from build123d import *

# Parameters (mm, degrees)
SKETCH2_W           = 250
SKETCH2_H           = 30
BOSS_EXTRUDE1_DEPTH = 10
SKETCH3_W           = 5
SKETCH3_H           = 30
BOSS_EXTRUDE2_DEPTH = 10
SKETCH4_W           = 150
SKETCH4_H           = 30
BOSS_EXTRUDE3_DEPTH = 6
FILLET1_R           = 15
FILLET8_R           = 25
CHAMFER1_SIZE       = 17
FILLET3_R           = 20
FILLET5_R           = 6
FILLET6_R           = 2
FILLET7_R           = 8
SKETCH7_W           = 24
SKETCH7_H           = 24
CUT_EXTRUDE1_DEPTH  = 3


with BuildPart() as part:
    # Sketch2 → Boss-Extrude1 (new body)
    with BuildSketch(Plane(origin=(-23.43534086, 72.126562752, 0), x_dir=(0.9510565162951534, 0.3090169943749482, 0), z_dir=(-0.3090169943749481, 0.9510565162951533, 0))):
        with Locations((33.98053096, 100)):
            Rectangle(SKETCH2_W, SKETCH2_H)
    extrude(amount=-BOSS_EXTRUDE1_DEPTH)

    # Sketch3 → Boss-Extrude2 (add)
    with BuildSketch(Plane(origin=(-23.43534086, 72.126562752, 0), x_dir=(0.9510565162951534, 0.3090169943749482, 0), z_dir=(-0.3090169943749481, 0.9510565162951533, 0))):
        with Locations((-88.51946904, 100)):
            Rectangle(SKETCH3_W, SKETCH3_H)
    extrude(amount=BOSS_EXTRUDE2_DEPTH)



with BuildPart() as body_2:
    # Sketch4 → Boss-Extrude3 (new body)
    with BuildSketch(Plane(origin=(0, 0, 0), x_dir=(1, 0, 0), z_dir=(0, 1, 0))):
        with Locations((55.854299018, 100)):
            Rectangle(SKETCH4_W, SKETCH4_H)
    extrude(amount=BOSS_EXTRUDE3_DEPTH)


with BuildPart() as part_1:
    add(part.part)

    add(body_2.part)  # Loft1 merges body 2
    # Sketch6 → Loft1 section 0
    with BuildSketch(Plane(origin=(-20.345170916, 62.615997589, 0), x_dir=(0.9510565162951534, 0.3090169943749482, 0), z_dir=(0.3090169943749481, -0.9510565162951533, 0))):
        with BuildLine():
            Line((158.98053096, -85), (148.98053096, -85))
            Line((148.98053096, -85), (148.98053096, -115))
            Line((148.98053096, -115), (158.98053096, -115))
            Line((158.98053096, -115), (158.98053096, -85))
        make_face()
    # Sketch5 → Loft1 section 1
    with BuildSketch(Plane(origin=(0, 6, 0), x_dir=(1, 0, 0), z_dir=(0, 1, 0))):
        with BuildLine():
            Line((130.854299018, 115), (120.854299018, 115))
            Line((120.854299018, 115), (120.854299018, 85))
            Line((120.854299018, 85), (130.854299018, 85))
            Line((130.854299018, 85), (130.854299018, 115))
        make_face()
    loft()

    # Fillet1
    fillet1_edges = [part_1.edges().sort_by_distance(p)[0] for p in [
        (130.854299018, 0, -100),
        (120.854299018, 6, -100),
    ]]
    fillet(fillet1_edges, radius=FILLET1_R)

    # Fillet8
    fillet8_edges = [part_1.edges().sort_by_distance(p)[0] for p in [
        (121.343733855, 108.653513487, -100),
    ]]
    fillet(fillet8_edges, radius=FILLET8_R)

    # Chamfer1
    # the kernel refuses this chamfer: 17 mm, written as the material it takes off along each edge
    with BuildSketch(Plane(origin=(127.764129074, 121.254248594, -41.281389205), x_dir=(-0.9591936310578489, -0.28275002765350715, 0), z_dir=(0, 0, -1))) as chamfer1_piece_1:
        Polygon((CHAMFER1_SIZE * 0.999621916911, -CHAMFER1_SIZE * 0.0274958766106), (-CHAMFER1_SIZE * 0.0274958766106, -CHAMFER1_SIZE * 0.999621916911), (0, 0), align=None)
    extrude(amount=117.437221591, mode=Mode.SUBTRACT)

    # Fillet3
    fillet3_edges = [part_1.edges().sort_by_distance(p)[0] for p in [
        (130.854299018, 106.188451977, -100),
        (111.596168297, 116.000959689, -100),
    ]]
    fillet(fillet3_edges, radius=FILLET3_R)

    # Fillet5
    fillet5_edges = [part_1.edges().sort_by_distance(p)[0] for p in [
        (-105.244717419, 45.545084972, -100),
    ]]
    fillet(fillet5_edges, radius=FILLET5_R)

    # Fillet6
    fillet6_edges = [part_1.edges().sort_by_distance(p)[0] for p in [
        (2.089489912, 80.420083013, -115),
        (-104.116423285, 47.759486891, -115),
        (-104.116423285, 47.759486891, -85),
        (-107.716853374, 53.153537102, -85),
        (-107.716853374, 53.153537102, -115),
        (-113.090169944, 53.510565163, -100),
        (-9.228059595, 66.228166023, -115),
        (-110.712528653, 54.283107649, -85),
        (-108.334887362, 55.055650135, -100),
        (-110.712528653, 54.283107649, -115),
        (43.389972522, 6, -85),
        (-19.145700982, 3, -115),
        (48.354299018, 0, -85),
        (-19.145700982, 3, -85),
        (43.389972522, 6, -115),
        (48.354299018, 0, -115),
        (126.460900735, 4.393398282, -115),
        (126.460900735, 4.393398282, -85),
        (116.506932566, 10.368143382, -85),
        (116.506932566, 10.368143382, -115),
        (121.052163557, 47.499886569, -115),
        (121.052163557, 47.499886569, -85),
        (-9.228059595, 66.228166023, -85),
        (110.921940595, 94.380821213, -115),
        (110.921940595, 94.380821213, -85),
        (-110, 44, -115),
        (-110, 44, -85),
        (130.854299018, 54.466218107, -115),
        (130.854299018, 54.466218107, -85),
        (119.455808519, 111.996272972, -85),
        (2.089489912, 80.420083013, -85),
        (111.466879946, 114.358195437, -85),
        (127.907102305, 104.382407509, -85),
        (119.455808519, 111.996272972, -115),
        (111.466879946, 114.358195437, -115),
        (127.907102305, 104.382407509, -115),
    ]]
    fillet(fillet6_edges, radius=FILLET6_R)

    # Fillet7
    # the kernel refuses this fillet: 8 mm, written as the material it takes off along each edge
    with BuildSketch(Plane(origin=(-101.773513881, 44.570022922, -85), x_dir=(-0.9510565162951534, -0.3090169943749482, 0), z_dir=(-0.3090169943749482, 0.9510565162951534, 0))) as fillet7_piece_1:
        with BuildLine():
            CenterArc((6, -2), 2, 0, 90)
            Line((8, -2), (8, 0))
            Line((8, 0), (6, 0))
        make_face()
    revolve(axis=Axis((-101.773513881, 44.570022922, -85), (0, 0, 1)), revolution_arc=90, mode=Mode.SUBTRACT)
    with BuildSketch(Plane(origin=(-101.773513881, 44.570022922, -115), x_dir=(0.3090169943749482, -0.9510565162951534, 0), z_dir=(0.9510565162951534, 0.3090169943749482, 0))) as fillet7_piece_2:
        with BuildLine():
            CenterArc((6, -2), 2, 0, 90)
            Line((8, -2), (8, 0))
            Line((8, 0), (6, 0))
        make_face()
    revolve(axis=Axis((-101.773513881, 44.570022922, -115), (0, 0, -1)), revolution_arc=90, mode=Mode.SUBTRACT)
    with BuildSketch(Plane(origin=(-106.909830056, 34.489434837, -115), x_dir=(0.9510565162951533, 0.3090169943749485, 0), z_dir=(0, 0, 1))) as fillet7_piece_3:
        with BuildLine():
            CenterArc((FILLET7_R, FILLET7_R), FILLET7_R, 180, 90)
            Line((0, FILLET7_R), (0, 0))
            Line((0, 0), (FILLET7_R, 0))
        make_face()
    extrude(amount=30, mode=Mode.SUBTRACT)

    # Sketch7 → Cut-Extrude1 (cut)
    with BuildSketch(Plane.XZ):
        with Locations((-13.956396798, -100)):
            Rectangle(SKETCH7_W, SKETCH7_H)
    extrude(amount=-CUT_EXTRUDE1_DEPTH, mode=Mode.SUBTRACT)


solid = part_1.part
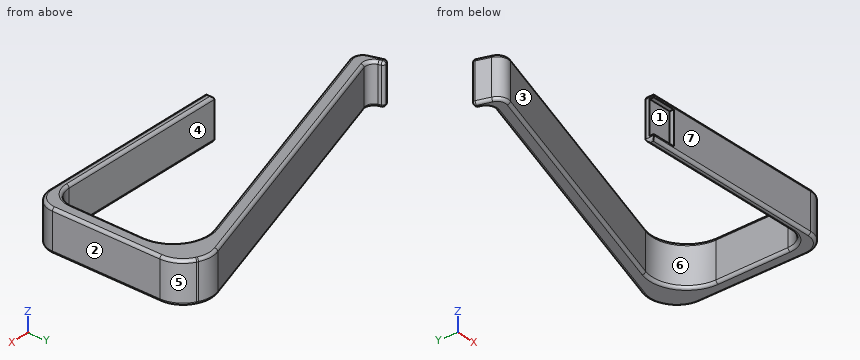
Source: CAD feature listing. Evaluate the final solid. Frame: model axes, mm. Face numbers are marked on the shaded views. A direction names the side the tool comes from. Give positions to 0.01 mm unless a question says otherwise; leave off trailing zeros. Use a Markdown table: item, result.
1) Ray query, line 1 along Y through (x, z) = (24.5, -100); line 2 along Y through (x, z) = (97, -88.5); line 3 along Y through (x, z) = (-97, -98.5). Return the intervals inside material, ascending. Write a range as [from, to].
Answer list:
| item | result |
|---|---|
| line 1 | [0, 6], [77.19, 87.7] |
| line 2 | [0, 6], [99.18, 111.26] |
| line 3 | [37.71, 48.22] |
2) Mould query, pull axis Y, two halves, no side actions, for the marked faces 5, 6 and 7. Classes: +Y half, -Y half, draft (parallel to the pull), parting line (faces both ways), or undercut.
Answer list:
| item | result |
|---|---|
| face 5 | +Y half |
| face 6 | undercut |
| face 7 | -Y half |
3) Contact query for flat-ended pins moving along their axis: P1, Ø3, axis at y = 54, z = -102.5, coming from the -X side; P2, Ø12, axis at y = 17, z = -97.5, coming from the -X side; P3, Ø10, axis at x = -51.5, z = -101.5, coming from the +Y side; P4, Ø12, axis at x = 32, y = 100.5, coming from the -Z side. Output: stop coordinate, or through.
Answer list:
| item | result |
|---|---|
| P1 | x = -112.55 |
| P2 | x = 117.11 |
| P3 | y = 64.63 |
| P4 | through |
4) Reachability of the marked faces 1, 2, 3 and 4 from +Z, -Z, +X, -X, +Y, -Y: full face, straight path, thin tool, end or side. Return the list, or none.
Answer list:
| item | result |
|---|---|
| face 1 | -X, -Y |
| face 2 | +Z, -Z, +X, +Y, -Y |
| face 3 | +Z, -Z |
| face 4 | +Z, -Z, -X |
